```python
from build123d import *

# Parameters (mm, degrees)
SKETCH1_W           = 120.396
SKETCH1_H           = 131.318
BOSS_EXTRUDE1_DEPTH = 34.544
SKETCH2_R           = 1.397
CUT_EXTRUDE1_DEPTH  = 35.544
SKETCH3_W           = 116.84
SKETCH3_H           = 30.48
BOSS_EXTRUDE2_DEPTH = 23.368
SKETCH4_R           = 5.715
CUT_EXTRUDE2_DEPTH  = 33.512
FILLET1_R           = 5.08


with BuildPart() as part:
    # Sketch1 → Boss-Extrude1 (new body)
    with BuildSketch(Plane(origin=(0, 0, 0), x_dir=(1, 0, 0), z_dir=(0, 1, 0))):
        with Locations((-83.235647386, 53.565832685)):
            Rectangle(SKETCH1_W, SKETCH1_H)
    extrude(amount=BOSS_EXTRUDE1_DEPTH)

    # Sketch2 → Cut-Extrude1 (cut, through all)
    with BuildSketch(Plane(origin=(0, 34.544, 0), x_dir=(1, 0, 0), z_dir=(0, 1, 0))):
        with Locations((-135.686647386, 103.730832685)):
            Circle(SKETCH2_R)
        with Locations((-30.686647386, 103.730832685)):
            Circle(SKETCH2_R)
        with Locations((-135.686647386, -1.269167315)):
            Circle(SKETCH2_R)
        with Locations((-30.686647328, -1.269167315)):
            Circle(SKETCH2_R)
    extrude(amount=-CUT_EXTRUDE1_DEPTH, mode=Mode.SUBTRACT)

    # Sketch3 → Boss-Extrude2 (add)
    with BuildSketch(Plane.XY.offset(12.093167315)):
        with Locations((-83.235647386, 17.272)):
            Rectangle(SKETCH3_W, SKETCH3_H)
    extrude(amount=BOSS_EXTRUDE2_DEPTH)

    # Sketch4 → Cut-Extrude2 (cut, through all)
    with BuildSketch(Plane(origin=(0, 32.512, 0), x_dir=(1, 0, 0), z_dir=(0, 1, 0))):
        with Locations((-128.320647386, -24.288198654)):
            Circle(SKETCH4_R)
        with Locations((-38.150647386, -23.777167315)):
            Circle(SKETCH4_R)
    extrude(amount=-CUT_EXTRUDE2_DEPTH, mode=Mode.SUBTRACT)

    # Fillet1
    fillet1_edges = [part.edges().sort_by_distance(p)[0] for p in [
        (-24.815647386, 17.272, 35.461167315),
        (-141.655647386, 17.272, 35.461167315),
        (-143.433647386, 17.272, -119.224832685),
        (-23.037647386, 17.272, -119.224832685),
    ]]
    fillet(fillet1_edges, radius=FILLET1_R)


solid = part.part
```
Design review of the part built by this model. Coordinates are the model's own, in mm. A direction names the side the tool comes from. Coordinates: 2 decimals unless noted, no trailing zeros. Order: outer loops, then holes, each group sorted by start corner. A loop starts at its lowest first (then second) coordinate and runs counter-clockwise, first axis right, second up. Notation, with made-up numbers: (61, 9.5) - (108, 9.5) arc R26 cw to (108, 43.5) - close; hole circle Ø7 at (-35, 83.5). An arc over 180 degrees is marked (long way). Answer in a Markdown table with one row per item.
(1) The part is to be moulded in two halves that separate along X. For faces 1 (the cylindrical face through (-122.87, 17.49, 22.57)), 2 (the flat face through (-143.434, 17, -50)), 3 (the cylindrical face through (-26.26, 17.49, 33.93)), say which applies: released by +X, released by -X, zero draft, split by the parting line, or undercut.
Checked values:
| item | result |
|---|---|
| face 1 | undercut |
| face 2 | released by -X |
| face 3 | released by +X |
(2) Consider section B-B on y = 10.5. State the section outline as (x, z) points (3 decimals).
Checked values:
| item | result |
|---|---|
| outline | (-143.434, -114.145) arc R5.08 ccw to (-138.354, -119.225) - (-28.118, -119.225) arc R5.08 ccw to (-23.038, -114.145) - (-23.038, 12.093) - (-24.816, 12.093) - (-24.816, 30.381) arc R5.08 ccw to (-29.896, 35.461) - (-136.576, 35.461) arc R5.08 ccw to (-141.656, 30.381) - (-141.656, 12.093) - (-143.434, 12.093) - close; hole circle Ø2.794 at (-135.687, -103.731); hole circle Ø2.794 at (-135.687, 1.269); hole circle Ø11.43 at (-128.321, 24.288); hole circle Ø11.43 at (-38.151, 23.777); hole circle Ø2.794 at (-30.687, -103.731); hole circle Ø2.794 at (-30.687, 1.269) |
(3) Consider section A-A on x = -119.5. State the section outline as (y, z) points.
Checked values:
| item | result |
|---|---|
| outline | (0, -119.22) - (34.54, -119.22) - (34.54, 12.09) - (32.51, 12.09) - (32.51, 35.46) - (2.03, 35.46) - (2.03, 12.09) - (0, 12.09) - close |
(4) For faces 4 (the flat face through (-24.816, 17, 21)), 5 (the flat face through (-84, 2.032, 24)), 6 (the flat face through (-84, 32.512, 24)), list the 3-axis set-ups (+Z, -Z, +X, -X, +Y, -Y) from which the entire face can be reached by the end or side of a thin tool; tool diameter is ignored.
Checked values:
| item | result |
|---|---|
| face 4 | +Z, +X, +Y, -Y |
| face 5 | +Z, +X, -X, -Y |
| face 6 | +Z, +X, -X, +Y |
(5) Wall thickness on line 1 along X through (y, z) = (11, -103.5); line 2 along Z through (x, y) = (-38.5, 22.5); line 3 along Y through (x, z) = (-108.5, 17): over which ranges is each line inside the solid? List them lowest first. Write a range as from..to.
Checked values:
| item | result |
|---|---|
| line 1 | -143.43..-137.06, -134.31..-32.06, -29.31..-23.04 |
| line 2 | -119.22..18.07, 29.48..35.46 |
| line 3 | 2.03..32.51 |
(6) Clearance check with flat-ended pins moving along their axes: pin 1 (11.5 mm diameter, centred on x = -70, z = 29, fed in from +Y); pin 2 (5.5 mm diameter, centred on y = 20, z = 25.5, fed in from -X); pin 3 (18.5 mm diameter, centred on x = -38.15, z = 23.78, fed in from -Y). State where each tip first meets the part, or that it passes through.
Checked values:
| item | result |
|---|---|
| pin 1 | y = 32.51 |
| pin 2 | x = -141.66 |
| pin 3 | y = 2.03 |
